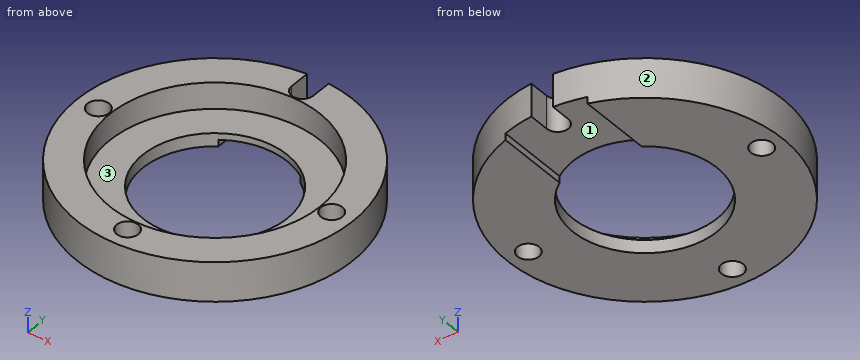
```python
from build123d import *

# Parameters (mm, degrees)
SKETCH_1_R          = 21
SKETCH_1_R_2        = 11
EXTRUDE_1_DEPTH     = 2
SKETCH_2_R          = 21
SKETCH_2_R_2        = 16
EXTRUDE_2_DEPTH     = 4
CUT_EXTRUDE_1_REACH = 32.299
SKETCH_3_R          = 1.65
CUT_EXTRUDE_2_REACH = 32.299
CUT_EXTRUDE_3_DEPTH = 1


with BuildPart() as part:
    # 草图1 → 凸台-拉伸1 (new body)
    with BuildSketch(Plane.XY):
        Circle(SKETCH_1_R)
        Circle(SKETCH_1_R_2, mode=Mode.SUBTRACT)
    extrude(amount=EXTRUDE_1_DEPTH)

    # 草图2 → 凸台-拉伸2 (add)
    with BuildSketch(Plane.XY.offset(2)):
        Circle(SKETCH_2_R)
        Circle(SKETCH_2_R_2, mode=Mode.SUBTRACT)
    extrude(amount=EXTRUDE_2_DEPTH)

    # 草图3 → 切除-拉伸1 (cut, up to next)
    with BuildSketch(Plane.XY.offset(6), mode=Mode.PRIVATE) as cut_extrude_1_sk1:
        with Locations((17.8, 0)):
            Circle(SKETCH_3_R)
    cut_extrude_1_tool1 = extrude(cut_extrude_1_sk1.sketch, amount=-CUT_EXTRUDE_1_REACH, mode=Mode.PRIVATE) & part.part
    # 草图3 → 切除-拉伸1 (cut, up to next)
    with BuildSketch(Plane.XY.offset(6), mode=Mode.PRIVATE) as cut_extrude_1_sk2:
        with Locations((0, -17.8)):
            Circle(SKETCH_3_R)
    cut_extrude_1_tool2 = extrude(cut_extrude_1_sk2.sketch, amount=-CUT_EXTRUDE_1_REACH, mode=Mode.PRIVATE) & part.part
    # 草图3 → 切除-拉伸1 (cut, up to next)
    with BuildSketch(Plane.XY.offset(6), mode=Mode.PRIVATE) as cut_extrude_1_sk3:
        with Locations((-17.8, 0)):
            Circle(SKETCH_3_R)
    cut_extrude_1_tool3 = extrude(cut_extrude_1_sk3.sketch, amount=-CUT_EXTRUDE_1_REACH, mode=Mode.PRIVATE) & part.part
    # 草图3 → 切除-拉伸1 (cut, up to next)
    with BuildSketch(Plane.XY.offset(6), mode=Mode.PRIVATE) as cut_extrude_1_sk4:
        with Locations((0, 17.8)):
            Circle(SKETCH_3_R)
    cut_extrude_1_tool4 = extrude(cut_extrude_1_sk4.sketch, amount=-CUT_EXTRUDE_1_REACH, mode=Mode.PRIVATE) & part.part
    add(cut_extrude_1_tool1.solids().sort_by_distance((17.8, 0, 6))[0], mode=Mode.SUBTRACT)
    add(cut_extrude_1_tool2.solids().sort_by_distance((0, -17.8, 6))[0], mode=Mode.SUBTRACT)
    add(cut_extrude_1_tool3.solids().sort_by_distance((-17.8, 0, 6))[0], mode=Mode.SUBTRACT)
    add(cut_extrude_1_tool4.solids().sort_by_distance((0, 17.8, 6))[0], mode=Mode.SUBTRACT)

    # 草图5 → 切除-拉伸2 (cut, up to next)
    with BuildSketch(Plane.XY.offset(6), mode=Mode.PRIVATE) as cut_extrude_2_sk1:
        with BuildLine():
            Line((-1.65, 17.8), (-1.65, 20.935078218))
            ThreePointArc((-1.65, 20.935078218), (0, 21), (1.65, 20.935078218))
            Line((1.65, 20.935078218), (1.65, 17.8))
            ThreePointArc((1.65, 17.8), (0, 19.45), (-1.65, 17.8))
        make_face()
    cut_extrude_2_tool1 = extrude(cut_extrude_2_sk1.sketch, amount=-CUT_EXTRUDE_2_REACH, mode=Mode.PRIVATE) & part.part
    add(cut_extrude_2_tool1.solids().sort_by_distance((0, 20.001216, 6))[0], mode=Mode.SUBTRACT)

    # 草图6 → 切除-拉伸3 (cut)
    with BuildSketch(Plane(origin=(0, 0, 0), x_dir=(-1, 0, 0), z_dir=(0, 0, -1))):
        with BuildLine():
            Line((-6.25, 9.051933495), (-6.25, 20.048378987))
            ThreePointArc((-6.25, 20.048378987), (0, 21), (6.25, 20.048378987))
            Line((6.25, 20.048378987), (6.25, 9.051933495))
            ThreePointArc((6.25, 9.051933495), (0, 11), (-6.25, 9.051933495))
        make_face()
    extrude(amount=-CUT_EXTRUDE_3_DEPTH, mode=Mode.SUBTRACT)


solid = part.part
```
Build history of the part. All positions in model axes, mm. Face numbers are marked on the shaded views. A direction names the side the tool comes from. Give positions to 0.01 mm unless a question says otherwise; leave off trailing zeros. Loops run counter-clockwise (first coordinate to the right, second up) from the corner with the lowest first, then second, coordinate; pieces in that order, holes last. Notation, with made-up numbers: (65.25, 33) -> (73.25, 33) arc R21 cw to (73.25, 43) -> close; hole circle Ø9 at (0, 64). An arc over 180 degrees is marked (long way). One line per question, with ' | ' between items. Start each with the question number.
1) Probe L1, parallel to Y at x = 0, z = 3.15; L2, parallel to Y at x = 0, z = 1.4; L3, parallel to Z at x = 12, y = 3.5. List the from-to ranges inside material, lowest first.
2) Cut at A-A (x = 0). Give the cut face in (y, z).
3) Pin check, flat tips, straight feed: pin 1 (1 mm diameter, centred on x = 3, z = 1.5, fed in from +Y); pin 2 (3.5 mm diameter, centred on y = 19.5, z = 4.5, fed in from +X); pin 3 (6 mm diameter, centred on x = 2.5, y = 13, fed in from -Z). Stop position of each tip, or through.
4) 3-axis set-ups, long thin cutter, end or side, ignore diameter. For the marked faces 1, 2 and 3: which of +Z, -Z, +X, -X, +Y, -Y reach the whole face in a straight line?
5) Cut at D-D (y = 8). Give the cut face in (x, z).
6) Cut at B-B (y = 0). Give the cut face in (x, z).
7) Cut at C-C (z = 3.55). Give the cut face in (x, y).
Return value:
1) L1: -21 to -19.45, -16.15 to -16, 16 to 16.15 | L2: -21 to -19.45, -16.15 to -11, 11 to 16.15 | L3: 0 to 2
2) outline: (-21, 0) -> (-19.45, 0) -> (-19.45, 6) -> (-21, 6) -> close; (-16.15, 0) -> (-11, 0) -> (-11, 2) -> (-16, 2) -> (-16, 6) -> (-16.15, 6) -> close; (11, 1) -> (16.15, 1) -> (16.15, 6) -> (16, 6) -> (16, 2) -> (11, 2) -> close
3) pin 1: y = 20.85 | pin 2: x = 11.22 | pin 3: z = 1
4) face 1: -Z, +Y | face 2: +Z, -Z | face 3: +Z
5) outline: (-19.42, 0) -> (-7.55, 0) -> (-7.55, 2) -> (-13.86, 2) -> (-13.86, 6) -> (-19.42, 6) -> close; (7.55, 0) -> (19.42, 0) -> (19.42, 6) -> (13.86, 6) -> (13.86, 2) -> (7.55, 2) -> close
6) outline: (-21, 0) -> (-19.45, 0) -> (-19.45, 6) -> (-21, 6) -> close; (-16.15, 0) -> (-11, 0) -> (-11, 2) -> (-16, 2) -> (-16, 6) -> (-16.15, 6) -> close; (11, 0) -> (16.15, 0) -> (16.15, 6) -> (16, 6) -> (16, 2) -> (11, 2) -> close; (19.45, 0) -> (21, 0) -> (21, 6) -> (19.45, 6) -> close
7) outline: (-1.65, 17.8) -> (-1.65, 20.94) arc R21 ccw (long way) to (1.65, 20.94) -> (1.65, 17.8) arc R1.65 cw to start; hole circle Ø3.3 at (-17.8, 0); hole circle Ø32 at (0, 0); hole circle Ø3.3 at (0, -17.8); hole circle Ø3.3 at (17.8, 0)
